Geometry check sheet. Reference: the model listing, model coordinates, mm. Face numbers are marked on the shaded views. A direction names the side the tool comes from. Give positions to 0.01 mm unless a question says otherwise; leave off trailing zeros. Write each loop counter-clockwise with the first axis right and the second up, starting at its lowest first coordinate (ties: lowest second). Pieces come first, ordered by that corner, then holes. Notation, with made-up numbers: M 6,44 L 61,44 A25 ccw 61,65 Z; hole C 1.25,40 d8. An arc over 180 degrees is marked long. One line per item, written item: value. Start each with the question number.
1. Tool access check on the marked faces 4 and 5. Record the directions out of +Z, -Z, +X, -X, +Y, -Y that give a thin tool (end or side, any length) a straight path to the whole face; none if there is none.
2. Scan lines: line 1 (Z direction, x = 3.5, y = 3.5); line 2 (X direction, y = 3, z = 2.5); line 3 (Y direction, x = -4.25, z = 1.25). Record each from-to range of solid material in increasing order.
3. Cross-section at B-B on z = 0. Record the cut outline in (x, y), then the cut area to 4 significant figures.
4. Gauge pin test, flat ends, axial feed: pin 1 (1.4 mm diameter, centred on x = 3.18, z = -3.18, fed in from +Y); pin 2 (6 mm diameter, centred on x = -3.5, y = 10, fed in from +Z); pin 3 (1.3 mm diameter, centred on x = -3.18, z = -3.18, fed in from -Y). Record the tip position at first contact, or that the pin passes through.
5. Release check for a two-part mould opening along Z. For the marked faces 1, 2 and 3 record: pulls with the +Z half, pulls with the -Z half, needs draft (parallel to the pull), parting line crosses it, or undercut.
6. Cross-section at A-A on y = 2.75. Record the cut outline in (x, z).
7. Cross-section at D-D on y = 0.5. Record the cut outline in (x, z), then the cut area to 3 significant figures.
from build123d import *

# Parameters (mm, degrees)
M2X0_4_TAPPED_HOLE1_D     = 1.6
M2X0_4_TAPPED_HOLE1_DEPTH = 5.2
M2X0_4_TAPPED_HOLE1_TIP   = 0.480688495
SKETCH7_W                 = 3
SKETCH7_H                 = 2
REVOLVE3_ANGLE            = 60
REVOLVE3_OTHER_WAY_ANGLE  = 10


with BuildPart() as part:
    # Sketch1 → Revolve1 (revolve)
    with BuildSketch(Plane.XY, mode=Mode.PRIVATE) as revolve1_sk:
        Polygon((-0.75, 0), (-7, 0), (-7, 12.5), (-0.75, 12.5), (-0.75, 16.6), (0, 16.6), (0, -0.9), (-0.75, -0.9), align=None)
    revolve(revolve1_sk.sketch.rotate(Axis((0, -74.460023863, 0), (0, 1, 0)), 270), axis=Axis((0, -74.460023863, 0), (0, 1, 0)))

    # M2x0.4 Tapped Hole1
    with Locations(Plane(origin=(0, 0, 0), x_dir=(-1, 0, 0), z_dir=(0, -1, 0))):
        with Locations((3.181980515, -3.181980515), (-3.181980515, -3.181980515), (-3.181980515, 3.181980515), (3.181980515, 3.181980515)):
            Hole(M2X0_4_TAPPED_HOLE1_D / 2, depth=M2X0_4_TAPPED_HOLE1_DEPTH)
            with Locations((0, 0, -(M2X0_4_TAPPED_HOLE1_DEPTH + M2X0_4_TAPPED_HOLE1_TIP / 2))):  # 118° drill point
                Cone(0, M2X0_4_TAPPED_HOLE1_D / 2, M2X0_4_TAPPED_HOLE1_TIP, mode=Mode.SUBTRACT)

    # Sketch7 → Revolve3 (revolve)
    with BuildSketch(Plane(origin=(0, 0, -7), x_dir=(-1, 0, 0), z_dir=(0, 0, -1))):
        with Locations((0, 1)):
            Rectangle(SKETCH7_W, SKETCH7_H)
    revolve(axis=Axis((-7, 6, -7), (1, 0, 0)), revolution_arc=REVOLVE3_ANGLE)

    # Sketch7 → Revolve3 other way (revolve)
    with BuildSketch(Plane(origin=(0, 0, -7), x_dir=(-1, 0, 0), z_dir=(0, 0, -1))):
        with Locations((0, 1)):
            Rectangle(SKETCH7_W, SKETCH7_H)
    revolve(axis=Axis((-7, 6, -7), (-1, 0, 0)), revolution_arc=REVOLVE3_OTHER_WAY_ANGLE)


solid = part.part
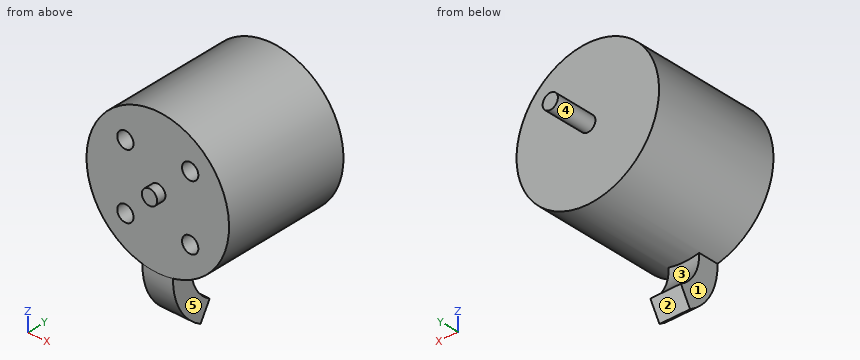
Report:
1. face 4: +Y
1. face 5: -Z, +X, +Y, -Y
2. line 1: z = -6.06 to -3.92, -2.45 to 2.45, 3.92 to 6.06
2. line 2: x = -6.54 to -3.6, -2.76 to 2.76, 3.6 to 6.54
2. line 3: y = 0 to 12.5
3. outline: M -7,0 L -0.75,0 L -0.75,-0.9 L 0.75,-0.9 L 0.75,0 L 7,0 L 7,12.5 L 0.75,12.5 L 0.75,16.6 L -0.75,16.6 L -0.75,12.5 L -7,12.5 Z
3. area: 182.5 mm^2
4. pin 1: stops at y = 12.5
4. pin 2: stops at z = 6.98
4. pin 3: stops at y = 5.29
5. face 1: needs draft
5. face 2: pulls with the -Z half
5. face 3: undercut
6. outline: C 0,0 d14; M -1.5,-12.04 L 1.5,-12.04 L 1.5,-9.33 L -1.5,-9.33 Z; hole C -3.18,-3.18 d1.6; hole C -3.18,3.18 d1.6; hole C 3.18,-3.18 d1.6; hole C 3.18,3.18 d1.6
7. outline: M -1.5,-9.4 L 1.5,-9.4 L 1.5,-6.84 A7 ccw long -1.5,-6.84 Z; hole C -3.18,-3.18 d1.6; hole C -3.18,3.18 d1.6; hole C 3.18,-3.18 d1.6; hole C 3.18,3.18 d1.6
7. area: 153 mm^2
